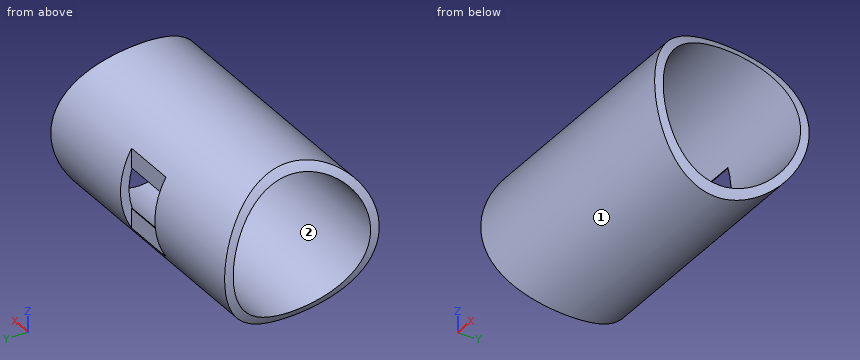
from build123d import *

# Parameters (mm, degrees)
BOSS_EXTRUDE1_DEPTH      = 101.15
BOSS_EXTRUDE1_DEPTH_BACK = 101.15
SKETCH1_R                = 57.15
SKETCH1_R_2              = 50.8
CUT_EXTRUDE3_DEPTH       = 130.474196271
CUT_EXTRUDE3_DEPTH_BACK  = 130.474196271
SKETCH3_W                = 40
SKETCH3_H                = 10
SKETCH5_W                = 40
SKETCH5_H                = 30
CUT_EXTRUDE5_DEPTH       = 18.15
CUT_EXTRUDE6_DEPTH       = 130.474196271
CUT_EXTRUDE6_DEPTH_BACK  = 130.474196271
SKETCH6_W                = 252.16572489
SKETCH6_H                = 244.887597008
SKETCH6_R                = 101.15


with BuildPart() as part:
    # Sketch1 → Boss-Extrude1 (new, two sides: drawn at the far end of the back side and taken through both)
    with BuildSketch(Plane(origin=(0, 0, 0), x_dir=(0, 0, -1), z_dir=(1, 0, 0)).offset(-BOSS_EXTRUDE1_DEPTH_BACK)):
        Circle(SKETCH1_R)
        Circle(SKETCH1_R_2, mode=Mode.SUBTRACT)
    extrude(amount=BOSS_EXTRUDE1_DEPTH + BOSS_EXTRUDE1_DEPTH_BACK)

    # Sketch3 → Cut-Extrude3 (cut, two sides: drawn at the far end of the back side and taken through both)
    with BuildSketch(Plane.XY.offset(-CUT_EXTRUDE3_DEPTH_BACK)):
        with Locations((0, 54)):
            Rectangle(SKETCH3_W, SKETCH3_H)
    extrude(amount=CUT_EXTRUDE3_DEPTH + CUT_EXTRUDE3_DEPTH_BACK, mode=Mode.SUBTRACT)

    # Sketch5 → Cut-Extrude5 (cut)
    with BuildSketch(Plane(origin=(0, 49, 0), x_dir=(1, 0, 0), z_dir=(0, 1, 0))):
        Rectangle(SKETCH5_W, SKETCH5_H)
    extrude(amount=-CUT_EXTRUDE5_DEPTH, mode=Mode.SUBTRACT)

    # Sketch6 → Cut-Extrude6 (cut, two sides: drawn at the far end of the back side and taken through both)
    with BuildSketch(Plane(origin=(0, 0, 0), x_dir=(1, 0, 0), z_dir=(0, 1, 0)).offset(-CUT_EXTRUDE6_DEPTH_BACK)):
        Rectangle(SKETCH6_W, SKETCH6_H)
        Circle(SKETCH6_R, mode=Mode.SUBTRACT)
    extrude(amount=CUT_EXTRUDE6_DEPTH + CUT_EXTRUDE6_DEPTH_BACK, mode=Mode.SUBTRACT)


solid = part.part
For this review, take the finished solid that the model builds, in its own axes (mm). Face numbers are marked on the shaded views. Round coordinates to 2 decimals unless told otherwise and drop trailing zeros. Loops run counter-clockwise (first coordinate to the right, second up) from the corner with the lowest first, then second, coordinate; pieces in that order, holes last. Notation, with made-up numbers: (32, 84) - (70, 84) arc R28 ccw to (70, 103) - close; hole circle Ø2 at (-35.75, -37). An arc over 180 degrees is marked (long way). Put each result on its own line as item: value. Start each with the question number.
1. Insertion check: P1, Ø1.5, axis at x = -29.5, z = -14.5, coming from the -Y side; P2, Ø10, axis at x = -78, y = 24.5, coming from the -Z side; P3, Ø8, axis at x = -76.5, z = 6, coming from the -Y side (3 decimals). Each pin has a flat end and moves straight along its axis. Give the tip position at first contact, or say it passes through.
2. For probe 1 along Y at (x, z) = (58, 0); probe 2 along Z at (x, y) = (20, -10.5), list the stretches that pass through material, from the lowest coordinate up. Write a range as [from, to].
3. Consider section B-B on y = 0. State the section outline as (x, z) points.
4. Consider section C-C on z = -32. State the section outline as (x, y) points, plus the area to 3 significant figures.
5. Mouldability with a two-part tool opening along Y and no side actions: class the marked faces 1 and 2 as +Y half, -Y half, draft (parallel to the pull), parting line (faces both ways), or undercut.
6. Consider section D-D on x = 5.5. State the section outline as (y, z) points, plus the area to 3 significant figures.
7. Consider section A-A on z = 0. State the section outline as (x, y) points, plus the area to 3 significant figures.
Result sheet:
1. P1: y = -55.47
1. P2: z = -53.72
1. P3: y = -57.115
2. probe 1: [-57.15, -50.8], [50.8, 57.15]
2. probe 2: [-56.18, -49.7], [49.7, 56.18]
3. outline: (-87.47, -50.8) arc R101.15 ccw to (-83.46, -57.15) - (83.46, -57.15) arc R101.15 ccw to (87.47, -50.8) - close; (-87.47, 50.8) - (87.47, 50.8) arc R101.15 ccw to (83.46, 57.15) - (-83.46, 57.15) arc R101.15 ccw to start
4. outline: (-95.95, -47.35) - (95.95, -47.35) - (95.95, -39.45) - (-95.95, -39.45) - close; (-95.95, 39.45) - (95.95, 39.45) - (95.95, 47.35) - (-95.95, 47.35) - close
4. area: 3,030 mm^2
5. face 1: parting line
5. face 2: undercut
6. outline: (48.53, -15) arc R50.8 cw (long way) to (48.53, 15) - (49, 15) - (49, 29.41) arc R57.15 ccw (long way) to (49, -29.41) - (49, -15) - close
6. area: 1,860 mm^2
7. outline: (-101.15, -57.15) - (101.15, -57.15) - (101.15, -50.8) - (-101.15, -50.8) - close; (-101.15, 50.8) - (-20, 50.8) - (-20, 57.15) - (-101.15, 57.15) - close; (20, 50.8) - (101.15, 50.8) - (101.15, 57.15) - (20, 57.15) - close
7. area: 2,320 mm^2
